Verification items for this drawing (mm, ordinates from the low corner). Coordinates: 2 decimals unless noted, no trailing zeros. Write each loop counter-clockwise with the first axis right and the second up, starting at its lowest first coordinate (ties: lowest second). Pieces come first, ordered by that corner, then holes. Notation, with made-up numbers: M 89,17.25 L 128,17.25 A28 cw 128,40.25 Z; hole C -7.75,9 d11. An arc over 180 degrees is marked long. Write each question's results on one line, items separated by ' | '.
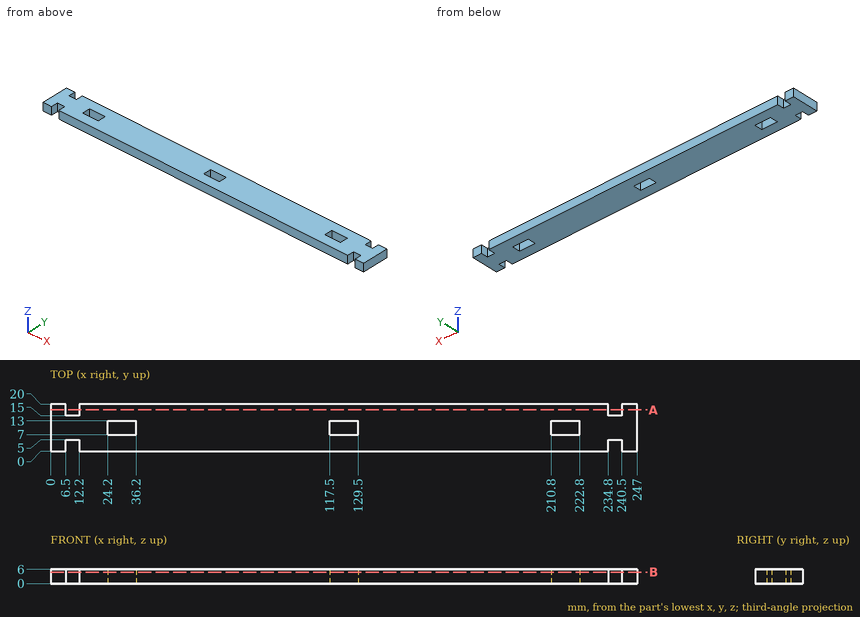
Q1. Depth check by flat-ended pin: P1, Ø1.7, axis at x = 238, z = 3, coming from the -Y side; P2, Ø3, axis at y = 10.5, z = 2.5, coming from the -X side; P3, Ø1.7, axis at x = 10.5, z = 4.5, coming from the +Y side. Enter the tip coordinate at first touch or a pass-through.
Geometry check:
P1: stops at y = 5 | P2: stops at x = 0 | P3: stops at y = 15
Q2. Scan lines: probe 1 along X at (y, z) = (16.25, 4.2); probe 2 along X at (y, z) = (10.75, 1.9); probe 3 along Y at (x, z) = (219.5, 2.8). Record each from-to range of solid material in increasing order.
Geometry check:
probe 1: x = 0 to 6.5, 12.2 to 234.8, 240.5 to 247 | probe 2: x = 0 to 24.2, 36.2 to 117.5, 129.5 to 210.8, 222.8 to 247 | probe 3: y = 0 to 7, 13 to 20
Q3. Sectioned sample at B-B on z = 4.9. Give the number of separate pieces and of enclosed holes in the cut face, and give its area (3 significant figures).
Geometry check:
separate pieces: 1 | enclosed holes: 3 | area: 4,610 mm2
Q4. Sectioned sample at A-A on y = 17.5. Record the cut outline in (x, z), and give its area (3 significant figures).
Geometry check:
outline: M 0,0 L 6.5,0 L 6.5,6 L 0,6 Z; M 12.2,0 L 234.8,0 L 234.8,6 L 12.2,6 Z; M 240.5,0 L 247,0 L 247,6 L 240.5,6 Z | area: 1,410 mm2
